```python
from build123d import *

# Parameters (mm, degrees)
F1_DEPTH      = 10
F1_DEPTH_BACK = 2
F3_R          = 1.9
F4_DEPTH      = 25
F2_R          = 3.1
F5_DEPTH      = 25
F6_SIZE       = 1


with BuildPart() as f1:
    # F0 (on Top) → F1 (new body, two sides)
    with BuildSketch(Plane.XY) as f1_sk:
        Polygon((8.5, 25), (0, 25), (-8.5, 25), (-8.5, 0), (-8.5, -25), (0, -25), (8.5, -25), (8.5, 0), align=None)
    extrude(amount=F1_DEPTH)
    extrude(f1_sk.sketch, amount=-F1_DEPTH_BACK)

    # F3 (on Top) → F4 (cut)
    with BuildSketch(Plane.XY):
        with Locations((3.5, 12.5)):
            Circle(F3_R)
        with Locations((-1.5, -12.5)):
            Circle(F3_R)
    extrude(amount=-F4_DEPTH, mode=Mode.SUBTRACT)

    # F2 (on Top) → F5 (cut)
    with BuildSketch(Plane.XY):
        with Locations((3.5, 12.5)):
            Circle(F2_R)
        with Locations((-1.5, -12.5)):
            Circle(F2_R)
    extrude(amount=F5_DEPTH, mode=Mode.SUBTRACT)

    # F6
    f6_edges = [f1.edges().sort_by_distance(p)[0] for p in [
        (-4.6, -12.5, 10),
        (0.4, 12.5, 10),
    ]]
    chamfer(f6_edges, length=F6_SIZE)


solid = f1.part
```
Read the model definition and answer for the solid it produces. Units are mm, in the model's axes. A direction names the side the tool comes from. Give positions to 0.01 mm unless a question says otherwise; leave off trailing zeros. Write each loop counter-clockwise with the first axis right and the second up, starting at its lowest first coordinate (ties: lowest second). Pieces come first, ordered by that corner, then holes. Notation, with made-up numbers: (-26, -25) - (0, -25) arc R14 cw to (0, -3) - close; hole circle Ø1 at (7.5, -24.75). An arc over 180 degrees is marked (long way). Write item = value, one per line. Start each with the question number.
Item 1: Find section B-B (y = -12.5). Give the vertices of the cut face in (x, z).
Item 2: Find section A-A (x = -1.5). Give the vertices of the cut face in (y, z).
Item 3: Find section C-C (z = 6). Give the vertices of the cut face in (x, y).
Item 4: This flat-tipped pin is pushed along its axis until it touches: P1, Ø1.9, axis at x = -0.5, y = -13.5, coming from the +Z side. Where does it stop, or does it pass through?
Item 5: A tool of negligible diameter and unlimited length cuts with its end or side. For faces 5 (the flat face through (-3, -14, 0)), 6 (the flat face through (-8.5, 0, 4)), from which of +Z, -Z, +X, -X, +Y, -Y can it reach the whole face along a straight path? Write none if from no direction.
Item 6: The mould has two halves that part along Y. Classify faces 1 (the flat face through (0, 25, 4)), 2 (the cylindrical face through (2.1, 13.784, -0.986)), 3 (the flat face through (0, 0, 10)), 4 (the flat face through (5, 14, 0)): +Y half, -Y half, draft (parallel to the pull), parting line (faces both ways), or undercut.
Item 7: Find the intervals of material crossed by probe 1 along Y at (x, z) = (-1.5, 5.5); probe 2 along Y at (x, z) = (3.5, 4.75); probe 3 along Y at (x, z) = (1, 7), in increasing order. Write a range as [from, to].
Response:
q1.outline = (-8.5, -2) - (-3.4, -2) - (-3.4, 0) - (-4.6, 0) - (-4.6, 9) - (-5.6, 10) - (-8.5, 10) - close; (0.4, -2) - (8.5, -2) - (8.5, 10) - (2.6, 10) - (1.6, 9) - (1.6, 0) - (0.4, 0) - close
q2.outline = (-25, -2) - (-14.4, -2) - (-14.4, 0) - (-15.6, 0) - (-15.6, 9) - (-16.6, 10) - (-25, 10) - close; (-10.6, -2) - (25, -2) - (25, 10) - (-8.4, 10) - (-9.4, 9) - (-9.4, 0) - (-10.6, 0) - close
q3.outline = (-8.5, -25) - (8.5, -25) - (8.5, 25) - (-8.5, 25) - close; hole circle Ø6.2 at (-1.5, -12.5); hole circle Ø6.2 at (3.5, 12.5)
q4.P1 = 0
q5.face_5 = +Z
q5.face_6 = +Z, -Z, -X, +Y, -Y
q6.face_1 = +Y half
q6.face_2 = undercut
q6.face_3 = draft
q6.face_4 = undercut
q7.probe_1 = [-25, -15.6], [-9.4, 25]
q7.probe_2 = [-25, 9.4], [15.6, 25]
q7.probe_3 = [-25, -14.33], [-10.67, 10.67], [14.33, 25]
